The figure shows three views and two pictorial views of one solid part (mm, origin at its lowest corner). Answer the questions. A direction names the side the tool comes from. Coordinates: 2 decimals unless noted, no trailing zeros. Order: outer loops, then holes, each group sorted by start corner. A loop starts at its lowest first (then second) coordinate and runs counter-clockwise, first axis right, second up. Notation, with made-up numbers: (82.5, 42) -> (114.5, 42) arc R33 ccw to (114.5, 74) -> close; hole circle Ø8 at (26, 73.25). An arc over 180 degrees is marked (long way). Write item = value, one per line. Start each with the question number.
Q1. The part is cut by section D-D, the plane z = 18.5. Determine the outline of the cut face in (x, y), plus the area to 3 significant figures.
Q2. The part is cut by section B-B, the plane z = 9. Determine the outline of the cut face in (x, y), plus the area to 3 significant figures.
Q3. Which of the six approach directions +Z, -Z, +X, -X, +Y, -Y give full straight-line access (tool end or side, diameter ignored) to the marked faces 4, 5 and 6?
Q4. The part is cut by section C-C, the plane y = 22.5. Determine the outline of the cut face in (x, z), plus the area to 3 significant figures.
Q5. Flat-ended cylindrical pins translate along their axes: pin 1 (3.5 mm diameter, centred on x = 1.5, z = 3.5, fed in from +Y); pin 2 (8 mm diameter, centred on x = 8.5, z = 5.5, fed in from -Y); pin 3 (3.5 mm diameter, centred on x = 18.5, z = 1.5, fed in from +Y); pin 4 (3.5 mm diameter, centred on x = 19, y = 25.5, fed in from -Z). Find the tip coordinate at first contact, or state that the pin passes through.
Q6. For a pull along Y with two mould halves and no side action, classify the marked faces 1, 2 and 3 as +Y half, -Y half, draft (parallel to the pull), parting line (faces both ways), or undercut.
Q7. The part is cut by section A-A, the plane x = 10. Determine the outline of the cut face in (y, z).
Q8. Straight lines are drawn through the part: L1, parallel to X at y = 21.5, z = 22.25; L2, parallel to Y at x = 12, z = 18; L3, parallel to Z at x = 6, y = 24.75. For each, find the intervals that lie inside material, in ascending order. Write a range as from..to.
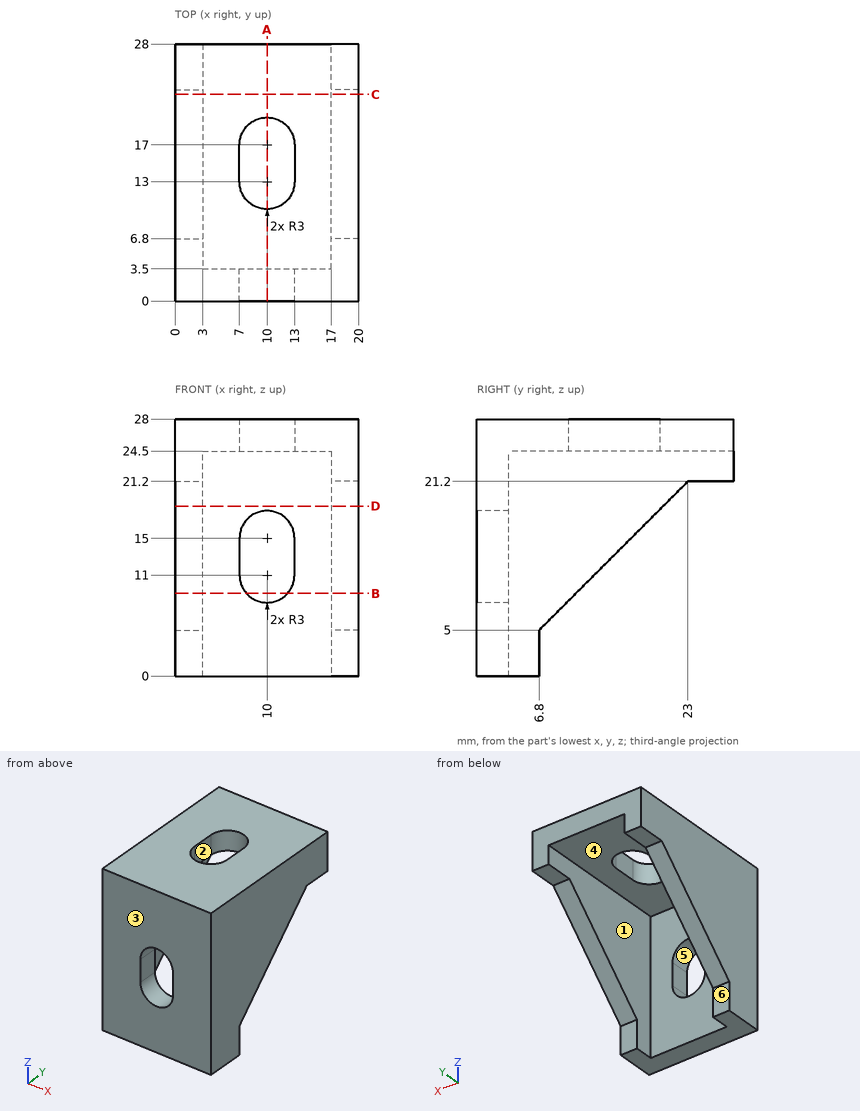
Model answer:
q1.outline = (0, 0) -> (20, 0) -> (20, 20.3) -> (17, 20.3) -> (17, 3.5) -> (3, 3.5) -> (3, 20.3) -> (0, 20.3) -> close
q1.area = 171 mm2
q2.outline = (0, 0) -> (7.76, 0) -> (7.76, 3.5) -> (3, 3.5) -> (3, 10.8) -> (0, 10.8) -> close; (12.24, 0) -> (20, 0) -> (20, 10.8) -> (17, 10.8) -> (17, 3.5) -> (12.24, 3.5) -> close
q2.area = 98.1 mm2
q3.face_4 = -Z, +Y
q3.face_5 = +Y, -Y
q3.face_6 = -Z, +X, -X, +Y
q4.outline = (0, 20.7) -> (3, 20.7) -> (3, 24.5) -> (17, 24.5) -> (17, 20.7) -> (20, 20.7) -> (20, 28) -> (0, 28) -> close
q4.area = 92.8 mm2
q5.pin_1 = 7.05
q5.pin_2 = 0
q5.pin_3 = 6.8
q5.pin_4 = 21.2
q6.face_1 = draft
q6.face_2 = undercut
q6.face_3 = -Y half
q7.outline = (0, 0) -> (3.5, 0) -> (3.5, 8) -> (0, 8) -> close; (0, 18) -> (3.5, 18) -> (3.5, 24.5) -> (10, 24.5) -> (10, 28) -> (0, 28) -> close; (20, 24.5) -> (28, 24.5) -> (28, 28) -> (20, 28) -> close
q8.L1 = 0..3, 17..20
q8.L2 = 0..3.5
q8.L3 = 24.5..28
